The listing builds one solid part. Answer for the finished solid, in the listing's coordinates (mm). Give positions to 0.01 mm unless a question says otherwise; leave off trailing zeros. Loops run counter-clockwise (first coordinate to the right, second up) from the corner with the lowest first, then second, coordinate; pieces in that order, holes last. Notation, with made-up numbers: (-29, 42) - (27, 42) arc R24 cw to (27, 52) - close; hole circle Ø10 at (-39.75, -24.5). An arc over 180 degrees is marked (long way). Answer in a Markdown table with one row per item. Add a question column.
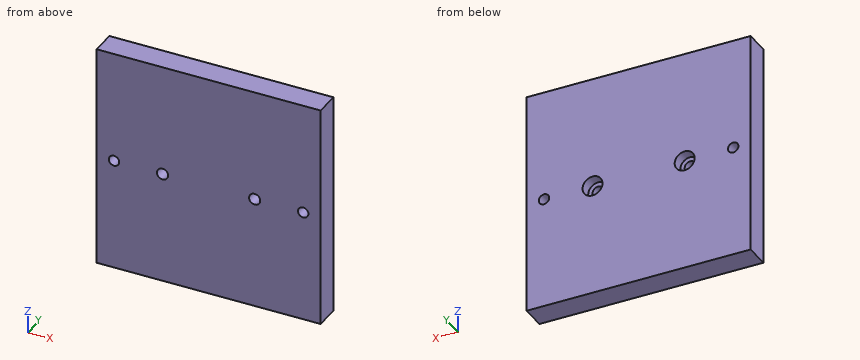
```python
from build123d import *

# Parameters (mm, degrees)
SKETCH1_W               = 90
SKETCH1_H               = 90
BOSS_EXTRUDE1_DEPTH     = 10
CUT_EXTRUDE1_DEPTH      = 95
CUT_EXTRUDE1_DEPTH_BACK = 74
SKETCH2_R               = 2.25
SKETCH2_3_R             = 4
SKETCH2_3_R_2           = 2.25
CUT_EXTRUDE2_DEPTH      = 4.4
M5_TAPPED_HOLE1_D       = 4.2


with BuildPart() as part:
    # Sketch1 → Boss-Extrude1 (new body)
    with BuildSketch(Plane(origin=(0, 0, 0), x_dir=(1, 0, 0), z_dir=(0, 1, 0))):
        with Locations((-60.460122699, -8.144171779)):
            Rectangle(SKETCH1_W, SKETCH1_H)
    extrude(amount=BOSS_EXTRUDE1_DEPTH)

    # Sketch2 → Cut-Extrude1 (cut, two sides: drawn at the far end of the back side and taken through both)
    with BuildSketch(Plane(origin=(0, 10, 0), x_dir=(1, 0, 0), z_dir=(0, 1, 0)).offset(-CUT_EXTRUDE1_DEPTH_BACK)):
        with Locations(Location((-78.960122699, -8.144171779, 0), (0, 0, 270))):
            Circle(SKETCH2_R)
        with Locations(Location((-41.960122699, -8.144171779, 0), (0, 0, 270))):
            Circle(SKETCH2_R)
    extrude(amount=CUT_EXTRUDE1_DEPTH + CUT_EXTRUDE1_DEPTH_BACK, mode=Mode.SUBTRACT)

    # Sketch2_3 → Cut-Extrude2 (cut)
    # profile 1 of 2: a face of its own
    with BuildSketch(Plane(origin=(0, 10, 0), x_dir=(1, 0, 0), z_dir=(0, 1, 0))):
        with Locations(Location((-78.960122699, -8.144171779, 0), (0, 0, 270))):
            Circle(SKETCH2_3_R)
        with Locations(Location((-78.960122699, -8.144171779, 0), (0, 0, 270))):
            Circle(SKETCH2_3_R_2, mode=Mode.SUBTRACT)
    # profile 2 of 2: a face of its own
    with BuildSketch(Plane(origin=(0, 10, 0), x_dir=(1, 0, 0), z_dir=(0, 1, 0))):
        with Locations(Location((-41.960122699, -8.144171779, 0), (0, 0, 270))):
            Circle(SKETCH2_3_R)
        with Locations(Location((-41.960122699, -8.144171779, 0), (0, 0, 270))):
            Circle(SKETCH2_3_R_2, mode=Mode.SUBTRACT)
    extrude(amount=-CUT_EXTRUDE2_DEPTH, mode=Mode.SUBTRACT)

    # M5 Tapped Hole1 (through all)
    with Locations(Plane(origin=(0, 10, 0), x_dir=(1, 0, 0), z_dir=(0, 1, 0))):
        with Locations((-98.460122699, -8.144171779), (-22.460122699, -8.144171779)):
            Hole(M5_TAPPED_HOLE1_D / 2)


solid = part.part
```
(1) A cutting plane is placed at A-A on y = 8.5. Determine the outline of the cut face in (x, z).
(2) Find the intervals of material crossed by line 1 along Z through (x, y) = (-21, 7.75); line 2 along Z through (x, y) = (-22, 8.5), in increasing order. Write a range as [from, to].
(3) Given pin 1 Ø7 at (x, z) = (-41.96, 8.14) entering from +Y; pin 2 Ø6.5 at (x, z) = (-79, 7) entering from +Y; pin 3 Ø2.5 at (x, z) = (-98.46, 8.14) entering from -Y, each flat-ended and moving along its own axis, determine where each tip first touches the part or whether it passes through.
Evaluation:
| question | item | result |
|---|---|---|
| 1 | outline | (-105.46, -36.86) - (-15.46, -36.86) - (-15.46, 53.14) - (-105.46, 53.14) - close; hole circle Ø4.2 at (-98.46, 8.14); hole circle Ø8 at (-78.96, 8.14); hole circle Ø8 at (-41.96, 8.14); hole circle Ø4.2 at (-22.46, 8.14) |
| 2 | line 1 | z = [-36.86, 6.63], [9.65, 53.14] |
| 2 | line 2 | z = [-36.86, 6.1], [10.19, 53.14] |
| 3 | pin 1 | stops at y = 5.6 |
| 3 | pin 2 | stops at y = 10 |
| 3 | pin 3 | passes through |
